from build123d import *

# Parameters (mm, degrees)
SKETCH1_W           = 2.5
SKETCH1_H           = 2.5
BOSS_EXTRUDE1_DEPTH = 1.5
SKETCH2_R           = 0.4953
BOSS_EXTRUDE2_DEPTH = 2.25
CHAMFER1_SIZE       = 0.5
CHAMFER1_SIZE2      = 0.288675135
CHAMFER2_SIZE       = 0.5
SKETCH4_R           = 0.4953
BOSS_EXTRUDE3_DEPTH = 3.5
CHAMFER3_SIZE       = 0.5
CHAMFER3_SIZE2      = 0.288675135


with BuildPart() as part:
    # Sketch1 → Boss-Extrude1 (new body, symmetric)
    with BuildSketch(Plane(origin=(0, 0, 0), x_dir=(1, 0, 0), z_dir=(0, 1, 0))):
        Rectangle(SKETCH1_W, SKETCH1_H)
    extrude(amount=BOSS_EXTRUDE1_DEPTH, both=True)

    # Sketch2 → Boss-Extrude2 (add)
    with BuildSketch(Plane(origin=(0, 1.5, 0), x_dir=(1, 0, 0), z_dir=(0, 1, 0))):
        Circle(SKETCH2_R)
    extrude(amount=BOSS_EXTRUDE2_DEPTH)

    # Chamfer1
    chamfer1_edges = [part.edges().sort_by_distance(p)[0] for p in [
        (-0.4953, 3.75, 0),
    ]]
    chamfer1_side = [part.faces().sort_by_distance(p)[0] for p in [
        (-0.4953, 2.625, 0),
    ]]
    chamfer(chamfer1_edges, length=CHAMFER1_SIZE, length2=CHAMFER1_SIZE2, reference=chamfer1_side[0])

    # Chamfer2
    chamfer2_edges = [part.edges().sort_by_distance(p)[0] for p in [
        (-1.25, 0, 1.25),
        (-1.25, 0, -1.25),
        (1.25, 0, -1.25),
        (1.25, 0, 1.25),
    ]]
    chamfer(chamfer2_edges, length=CHAMFER2_SIZE)

    # Sketch4 → Boss-Extrude3 (add)
    with BuildSketch(Plane.XZ.offset(1.5)):
        Circle(SKETCH4_R)
    extrude(amount=BOSS_EXTRUDE3_DEPTH)

    # Chamfer3
    chamfer3_edges = [part.edges().sort_by_distance(p)[0] for p in [
        (-0.4953, -5, 0),
    ]]
    chamfer3_side = [part.faces().sort_by_distance(p)[0] for p in [
        (-0.4953, -3.25, 0),
    ]]
    chamfer(chamfer3_edges, length=CHAMFER3_SIZE, length2=CHAMFER3_SIZE2, reference=chamfer3_side[0])


solid = part.part
Verification items for the finished model (mm, model axes). A direction names the side the tool comes from. Coordinates: 2 decimals unless noted, no trailing zeros. Write each loop counter-clockwise with the first axis right and the second up, starting at its lowest first coordinate (ties: lowest second). Pieces come first, ordered by that corner, then holes. Notation, with made-up numbers: M 62,-21 L 74,-21 A23 ccw 74,-10 Z; hole C 55,33.25 d5. An arc over 180 degrees is marked long. Use CSV: the item, a comma, the result in double quotes.
Q1. Go/stop test with a flat-tipped pin: P1, Ø1, axis at y = 2.5, z = -0.5, coming from the +X side. Record where the tip stops, or that it passes through.
Computed values:
P1,"x = 0.5"
Q2. Section check B-B, the plane x = 0. Enter the section's corners in (y, z).
Computed values:
outline,"M -5,-0.21 L -4.5,-0.5 L -1.5,-0.5 L -1.5,-1.25 L 1.5,-1.25 L 1.5,-0.5 L 3.25,-0.5 L 3.75,-0.21 L 3.75,0.21 L 3.25,0.5 L 1.5,0.5 L 1.5,1.25 L -1.5,1.25 L -1.5,0.5 L -4.5,0.5 L -5,0.21 Z"
Q3. Thickness scan on line 1 along Z through (x, y) = (0, -4.25); line 2 along Y through (x, z) = (1.1, -0.2); line 3 along X through (y, z) = (-4, 0.05). Record the ranges inside material, lowest first. Write a range as [from, to].
Computed values:
line 1,"[-0.5, 0.5]"
line 2,"[-1.5, 1.5]"
line 3,"[-0.49, 0.49]"
Q4. Section check A-A, the plane y = -1. Enter the section's corners in (x, z).
Computed values:
outline,"M -1.25,-0.75 L -0.75,-1.25 L 0.75,-1.25 L 1.25,-0.75 L 1.25,0.75 L 0.75,1.25 L -0.75,1.25 L -1.25,0.75 Z"
Q5. Section check D-D, the plane y = -3.75. Enter the section's corners in (x, z).
Computed values:
outline,"C 0,0 d0.99"
Q6. Set-up check for faces 1 (the cylindrical face through (-0.06, -2.98, 0.49)), 2 (the flat face through (1, 1.5, 0)), 3 (the flat face through (-1.25, 0, 0)): record each of +Z, -Z, +X, -X, +Y, -Y from which the full face is reachable in a straight line by a thin tool's end or side.
Computed values:
face 1,"-Y"
face 2,"+Y"
face 3,"+Z, -Z, -X, +Y, -Y"
Q7. Section check C-C, the plane z = 0. Enter the section's corners in (x, y), and give its area (3 significant figures).
Computed values:
outline,"M -1.25,-1.5 L -0.5,-1.5 L -0.5,-4.5 L -0.21,-5 L 0.21,-5 L 0.5,-4.5 L 0.5,-1.5 L 1.25,-1.5 L 1.25,1.5 L 0.5,1.5 L 0.5,3.25 L 0.21,3.75 L -0.21,3.75 L -0.5,3.25 L -0.5,1.5 L -1.25,1.5 Z"
area,"12.9 mm²"
